Input: part model. Units: mm. Frame: model coordinates. A direction names the side the tool comes from. Give positions to 0.01 mm unless a question says otherwise; leave off trailing zeros. Order: outer loops, then holes, each group sorted by start corner. A loop starts at its lowest first (then second) coordinate and runs counter-clockwise, first axis right, second up. Notation, with made-up numbers: (60.5, 58) - (67.5, 58) arc R6 cw to (67.5, 65) - close; hole circle Ø10 at (26.5, 12.5). An arc over 180 degrees is marked (long way). Use a Markdown table: item, result.
from build123d import *

# Parameters (mm, degrees)
F1_DEPTH = 16
F2_R     = 2.1
F3_DEPTH = 3
F4_SIZE  = 4
F6_DEPTH = 2.5
F7_SIZE  = 1.49999


# Not quite as in the source:
# - a fillet or chamfer is up to 0.001 mm smaller than in the source, because OpenCascade refuses the exact size


with BuildPart() as f1:
    # F0 (on Front) → F1 (new body)
    with BuildSketch(Plane.XZ):
        with BuildLine():
            ThreePointArc((-5.7283718128, -4.9945726919), (-6.9180471398, 3.1465256666), (0, 7.6))
            Line((0, 7.6), (0, 10.6))
            ThreePointArc((0, 10.6), (-8.4743731332, 6.367495583), (-10.1812327348, -2.95))
            Line((-10.1812327348, -2.95), (-20, -2.95))
            Line((-20, -2.95), (-20, -5.95))
            Line((-20, -5.95), (-5.7283718128, -5.95))
            Line((-5.7283718128, -5.95), (-5.7283718128, -4.9945726919))
        make_face()
        with BuildLine():
            Line((0, 10.6), (0, 7.6))
            ThreePointArc((0, 7.6), (6.9180471398, 3.1465256666), (5.7283718128, -4.9945726919))
            Line((5.7283718128, -4.9945726919), (5.7283718128, -5.95))
            Line((5.7283718128, -5.95), (20, -5.95))
            Line((20, -5.95), (20, -2.95))
            Line((20, -2.95), (10.1812327348, -2.95))
            ThreePointArc((10.1812327348, -2.95), (8.4743731332, 6.367495583), (0, 10.6))
        make_face()
    extrude(amount=F1_DEPTH)

    # F2 (on face) → F3 (cut, through all)
    with BuildSketch(Plane.XY.offset(-2.95)):
        with Locations((-14, -10.5)):
            Circle(F2_R)
        with Locations((14, -10.5)):
            Circle(F2_R)
    extrude(amount=-F3_DEPTH, mode=Mode.SUBTRACT)

    # F4
    f4_edges = [f1.edges().sort_by_distance(p)[0] for p in [
        (-20, -16, -4.45),
        (20, -16, -4.45),
    ]]
    chamfer(f4_edges, length=F4_SIZE)

    # F5 (on face) → F6 (join)
    with BuildSketch(Plane.XZ.offset(16)):
        with BuildLine():
            Line((5.7283718128, -2.0966059178), (5.7283718128, -4.9945726919))
            ThreePointArc((5.7283718128, -4.9945726919), (0, 7.6), (-5.7283718128, -4.9945726919))
            Line((-5.7283718128, -4.9945726919), (-5.7283718128, -2.0966059178))
            ThreePointArc((-5.7283718128, -2.0966059178), (0, 6.1), (5.7283718128, -2.0966059178))
        make_face()
    extrude(amount=-F6_DEPTH)

    # F7 (size 1.5 in the source; OpenCascade refuses exactly that, so slightly less here)
    f7_edges = [f1.edges().sort_by_distance(p)[0] for p in [
        (0, -13.5, 6.1),
    ]]
    chamfer(f7_edges, length=F7_SIZE)

    # F8: F1 across plane


with BuildPart() as f1_1:
    add(f1.part)
    add(f1.part.mirror(Plane.XZ))


solid = f1_1.part
1. Material intervals for line 1 along Y through (x, z) = (-14, -4.05); line 2 along X through (y, z) = (10.5, -4.8); line 3 along X through (y, z) = (6.5, 0), sorted ascending.
Response:
| item | result |
|---|---|
| line 1 | y = -16 to -12.6, -8.4 to 8.4, 12.6 to 16 |
| line 2 | x = -20 to -16.1, -11.9 to -5.89, 5.89 to 11.9, 16.1 to 20 |
| line 3 | x = -10.6 to -7.6, 7.6 to 10.6 |
2. Section query D-D (z = 8.5). Return loops of the section in (x, y).
Response:
| item | result |
|---|---|
| outline | (-6.33, -16) - (6.33, -16) - (6.33, 16) - (-6.33, 16) - close |
3. Set-up query: faces 4 (the face through (-0.164, 15.507, 6.098)), 5 (the face through (-5.728, 0.1, -5.2)), 6 (the face through (-0.203, 14.76, 6.336)). Return all of +Z, -Z, +X, -X, +Y, -Y with unobstructed straight access to the full face (end or side cutting, diameter ignored); none if empty.
Response:
| item | result |
|---|---|
| face 4 | +Y, -Y |
| face 5 | -Z, +Y, -Y |
| face 6 | none |
4. Section query C-C (y = 2.5). Return loops of the section in (x, z), then the cut area to 3 significant figures.
Response:
| item | result |
|---|---|
| outline | (-20, -5.95) - (-5.73, -5.95) - (-5.73, -4.99) arc R7.6 cw (long way) to (5.73, -4.99) - (5.73, -5.95) - (20, -5.95) - (20, -2.95) - (10.18, -2.95) arc R10.6 ccw (long way) to (-10.18, -2.95) - (-20, -2.95) - close |
| area | 187 mm^2 |
5. Pin query (flat end, axial travel): pin 1 (1 mm diameter, centred on x = -10.5, z = 4, fed in from -Y); pin 2 (11 mm diameter, centred on x = -16.5, y = -5.5, fed in from +Z); pin 3 (3 mm diameter, centred on y = -3.5, z = 3.5, fed in from +X); pin 4 (6.5 mm diameter, centred on x = 14, y = 10.5, fed in from -Z). Return the tip coordinate at first contact, or that it passes through.
Response:
| item | result |
|---|---|
| pin 1 | passes through |
| pin 2 | stops at z = -2.95 |
| pin 3 | stops at x = 10.41 |
| pin 4 | stops at z = -5.95 |
6. Section query B-B (y = 10.5). Return loops of the section in (x, z), then the cut area to 3 significant figures.
Response:
| item | result |
|---|---|
| outline | (-20, -5.95) - (-16.1, -5.95) - (-16.1, -2.95) - (-20, -2.95) - close; (-11.9, -5.95) - (-5.73, -5.95) - (-5.73, -4.99) arc R7.6 cw (long way) to (5.73, -4.99) - (5.73, -5.95) - (11.9, -5.95) - (11.9, -2.95) - (10.18, -2.95) arc R10.6 ccw (long way) to (-10.18, -2.95) - (-11.9, -2.95) - close; (16.1, -5.95) - (20, -5.95) - (20, -2.95) - (16.1, -2.95) - close |
| area | 161 mm^2 |
7. Section query A-A (x = -14). Return loops of the section in (y, z).
Response:
| item | result |
|---|---|
| outline | (-16, -5.95) - (-12.6, -5.95) - (-12.6, -2.95) - (-16, -2.95) - close; (-8.4, -5.95) - (8.4, -5.95) - (8.4, -2.95) - (-8.4, -2.95) - close; (12.6, -5.95) - (16, -5.95) - (16, -2.95) - (12.6, -2.95) - close |
8. Mould query, pull axis X, two halves, no side actions, for faces 1 (the face through (-18, -14, -4)), 2 (the face through (3, 16, 6)), 3 (the face through (-0.203, -14.76, 6.336)). Classes: pulls with the +X half, pulls with the -X half, needs draft (parallel to the pull), parting line crosses it, or undercut.
Response:
| item | result |
|---|---|
| face 1 | pulls with the -X half |
| face 2 | needs draft |
| face 3 | undercut |
